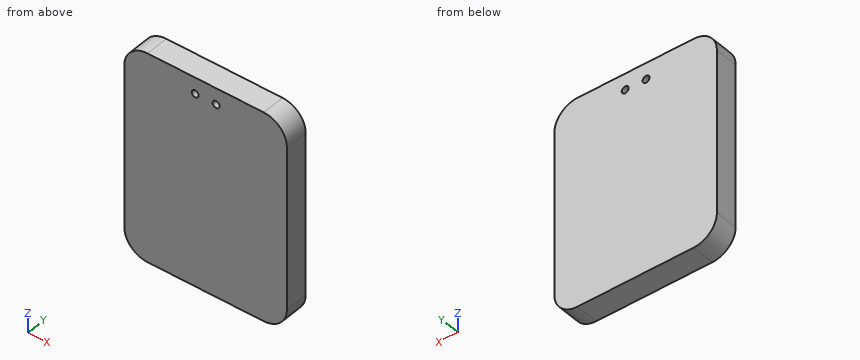
from build123d import *

# Parameters (mm, degrees)
SKETCH1_W           = 70
SKETCH1_H           = 90
BOSS_EXTRUDE1_DEPTH = 5
FILLET1_R           = 10
SKETCH2_R           = 1.5
CUT_EXTRUDE1_DEPTH  = 10


with BuildPart() as part:
    # Sketch1 → Boss-Extrude1 (new, symmetric)
    with BuildSketch(Plane(origin=(0, 0, 0), x_dir=(1, 0, 0), z_dir=(0, 1, 0))):
        Rectangle(SKETCH1_W, SKETCH1_H)
    extrude(amount=BOSS_EXTRUDE1_DEPTH, both=True)

    # Fillet1
    fillet1_edges = [part.edges().sort_by_distance(p)[0] for p in [
        (-35, 0, -45),
        (35, 0, -45),
        (35, 0, 45),
        (-35, 0, 45),
    ]]
    fillet(fillet1_edges, radius=FILLET1_R)

    # Sketch2 → Cut-Extrude1 (cut)
    with BuildSketch(Plane(origin=(0, 5, 0), x_dir=(1, 0, 0), z_dir=(0, 1, 0))):
        with Locations(Location((-4.5, -38, 0), (0, 0, 270))):
            Circle(SKETCH2_R)
        with Locations(Location((4.5, -38, 0), (0, 0, 270))):
            Circle(SKETCH2_R)
    extrude(amount=-CUT_EXTRUDE1_DEPTH, mode=Mode.SUBTRACT)


solid = part.part
Could you check a few things on this model? Use its own coordinates, in mm. Coordinates: 2 decimals unless noted, no trailing zeros. Loops run counter-clockwise (first coordinate to the right, second up) from the corner with the lowest first, then second, coordinate; pieces in that order, holes last.
1. Imagine slicing it at B-B (x = -4.5). Please give me the cut outline in (y, z), and give its area (3 significant figures).
2. I need wall thicknesses on L1, parallel to X at y = 0.5, z = 38; L2, parallel to Z at x = -4, y = 0; L3, parallel to X at y = 0.25, z = -39.5. Which ranges of each line are inside material? Lowest first, please.
3. Imagine slicing it at A-A (y = -3). Please give me the cut outline in (x, z).
4. Imagine slicing it at C-C (z = 38). Please give me the cut outline in (x, y), and give its area (3 significant figures).
Computed values:
1. outline: (-5, -45) - (5, -45) - (5, 36.5) - (-5, 36.5) - close; (-5, 39.5) - (5, 39.5) - (5, 45) - (-5, 45) - close
1. area: 870 mm2
2. L1: x = -34.54 to -6, -3 to 3, 6 to 34.54
2. L2: z = -45 to 36.59, 39.41 to 45
2. L3: x = -33.93 to 33.93
3. outline: (-35, -35) arc R10 ccw to (-25, -45) - (25, -45) arc R10 ccw to (35, -35) - (35, 35) arc R10 ccw to (25, 45) - (-25, 45) arc R10 ccw to (-35, 35) - close; hole circle Ø3 at (-4.5, 38); hole circle Ø3 at (4.5, 38)
4. outline: (-34.54, -5) - (-6, -5) - (-6, 5) - (-34.54, 5) - close; (-3, -5) - (3, -5) - (3, 5) - (-3, 5) - close; (6, -5) - (34.54, -5) - (34.54, 5) - (6, 5) - close
4. area: 631 mm2
